```python
from build123d import *

# Parameters (mm, degrees)
BOSS_EXTRUDE1_DEPTH = 25.4
SKETCH9_R           = 5.715
CUT_EXTRUDE1_DEPTH  = 26.4
FILLET9_R           = 2.54
FILLET10_R          = 1.27


with BuildPart() as part:
    # Sketch2 → Boss-Extrude1 (new body)
    with BuildSketch(Plane.XY):
        Polygon((0, 0), (0, 92.075), (18.075, 92.075), (38.575, 92.075), (57.15, 92.075), (57.15, 76.835), (88.9, 76.835), (88.9, 0), align=None)
    extrude(amount=BOSS_EXTRUDE1_DEPTH)

    # Sketch9 → Cut-Extrude1 (cut, through all)
    with BuildSketch(Plane.XY.offset(25.4)):
        with Locations((28.566361876, 80.645)):
            Circle(SKETCH9_R)
    extrude(amount=-CUT_EXTRUDE1_DEPTH, mode=Mode.SUBTRACT)

    # Fillet9
    fillet9_edges = [part.edges().sort_by_distance(p)[0] for p in [
        (57.15, 84.455, 0),
        (73.025, 76.835, 0),
        (88.9, 38.4175, 0),
        (73.025, 76.835, 25.4),
        (0, 92.075, 12.7),
        (57.15, 92.075, 12.7),
        (88.9, 76.835, 12.7),
        (57.15, 84.455, 25.4),
        (28.575, 92.075, 25.4),
        (0, 46.0375, 25.4),
        (0, 46.0375, 0),
        (88.9, 38.4175, 25.4),
        (28.575, 92.075, 0),
    ]]
    fillet(fillet9_edges, radius=FILLET9_R)

    # Fillet10
    fillet10_edges = [part.edges().sort_by_distance(p)[0] for p in [
        (22.851361876, 80.645, 0),
        (22.851361876, 80.645, 25.4),
    ]]
    fillet(fillet10_edges, radius=FILLET10_R)


solid = part.part
```
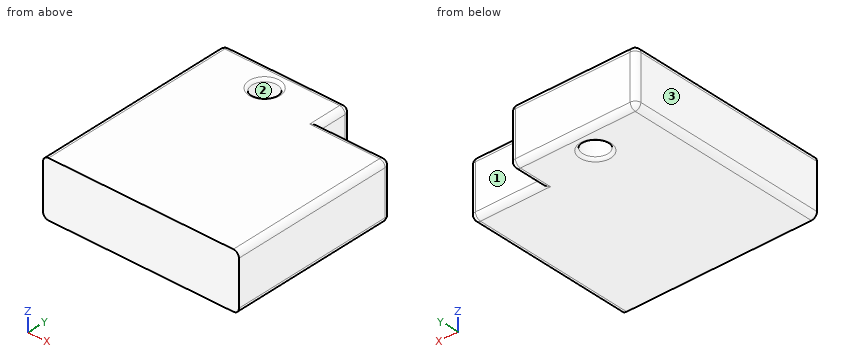
The listing builds one solid part. Answer for the finished solid, in the listing's coordinates (mm). Face numbers are marked on the shaded views. Give positions to 0.01 mm unless a question says otherwise; leave off trailing zeros. Order: outer loops, then holes, each group sorted by start corner. A loop starts at its lowest first (then second) coordinate and runs counter-clockwise, first axis right, second up. Notation, with made-up numbers: (29.5, -31.5) - (82.5, -31.5) arc R30 cw to (82.5, -1.5) - close; hole circle Ø5 at (51.5, 62). An arc over 180 degrees is marked (long way). Answer in a Markdown table with one row per item. Add a question column.
Q1. The part is cut by section A-A (z = 12.5). Determine the outline of the cut face in (x, y) (3 decimals), then the cut area to 3 significant figures.
Q2. For a pull along X with two mould halves and no side action, classify the marked faces 1, 2 and 3 as released by +X, released by -X, zero draft, split by the parting line, or undercut.
Q3. Given P1, Ø10, axis at y = 85, z = 14, coming from the +X side; P2, Ø12, axis at x = 66.5, z = 10.5, coming from the +Y side (3 decimals), each flat-ended and moving along its own axis, determine where each tip first touches the part or whether it passes through.
Q4. Find the intervals of material crossed by line 1 along Y through (x, z) = (70.5, 6.75) (3 decimals); line 2 along X through (y, z) = (84, 9.75); line 3 along Y through (x, z) = (56, 15), in increasing order. Write a range as [from, to].
Q5. The part is cut by section B-B (x = 75.5). Determine the outline of the cut face in (y, z) (3 decimals).
Determined:
| question | item | result |
|---|---|---|
| 1 | outline | (0, 0) - (88.9, 0) - (88.9, 74.295) arc R2.54 ccw to (86.36, 76.835) - (57.15, 76.835) - (57.15, 89.535) arc R2.54 ccw to (54.61, 92.075) - (2.54, 92.075) arc R2.54 ccw to (0, 89.535) - close; hole circle Ø11.43 at (28.566, 80.645) |
| 1 | area | 7,590 mm² |
| 2 | face 1 | zero draft |
| 2 | face 2 | undercut |
| 2 | face 3 | released by -X |
| 3 | P1 | stops at x = 57.15 |
| 3 | P2 | stops at y = 76.835 |
| 4 | line 1 | y = [0, 76.835] |
| 4 | line 2 | x = [0, 23.94], [33.19, 57.15] |
| 4 | line 3 | y = [0, 91.66] |
| 5 | outline | (0, 0) - (74.295, 0) arc R2.54 ccw to (76.835, 2.54) - (76.835, 22.86) arc R2.54 ccw to (74.295, 25.4) - (0, 25.4) - close |
